Verification items for the finished model (mm, model axes). A direction names the side the tool comes from. Coordinates: 2 decimals unless noted, no trailing zeros. Write each loop counter-clockwise with the first axis right and the second up, starting at its lowest first coordinate (ties: lowest second). Pieces come first, ordered by that corner, then holes. Notation, with made-up numbers: M 43,83.5 L 63,83.5 A11 cw 63,91.5 Z; hole C 2.25,-16 d5. An arc over 180 degrees is marked long. One line per item, written item: value.
Autodesk Inventor part; units mm, degrees
ref_plane "YZ Plane" through (0, 0, 0) normal (1, 0, 0) x (0, 1, 0)
ref_plane "XZ Plane" through (0, 0, 0) normal (0, 1, 0) x (-1, 0, 0)
ref_plane "XY Plane" through (0, 0, 0) normal (0, 0, 1) x (1, 0, 0)
sketch "Sketch1" plane through (0, 0, 0) normal (0, 0, 1) x (1, 0, 0)
  line L0 (0, 0) -> (40, 0)
  line L1 (40, 0) -> (40, -15)
  line L2 (40, -15) -> (0, -15)
  line L3 (0, -15) -> (0, 0)
  dimension "d0" = 40
  dimension "d1" = 15
extrude "Extrusion1" add sketch "Sketch1" along normal blind 5
sketch "Sketch2" plane through (0, 0, 5) normal (0, 0, 1) x (1, 0, 0)
  line L0 (40, 0) -> (0, 0)
  line L1 (5, 0) -> (35, 0)
  line L2 (35, 0) -> (35, -15)
  line L3 (35, -15) -> (5, -15)
  line L4 (5, -15) -> (5, 0)
  line L5 (0, 0) -> (0, -15)
  dimension "d4" = 30
  dimension "d5" = 15
  dimension "d6" = 5
extrude "Extrusion2" add sketch "Sketch2" along normal blind 3
fillet "Fillet1" radius 2 4 edges at (35, -7.5, 5) (35, -7.5, 8) (5, -7.5, 5) (5, -7.5, 8)
sketch "Sketch3" plane through (0, 0, 0) normal (0, 0, -1) x (-1, 0, 0)
  line L0 (0, 0) -> (0, -15)
  line L1 (-40, 0) -> (0, 0)
  line L2 (0, -15) -> (-5, -15)
  line L3 (-5, -15) -> (-5, 0)
  line L4 (-5, 0) -> (0, 0)
  line L5 (0, 0) -> (0, -15)
  line L6 (-40, -15) -> (-40, 0)
  line L7 (0, -15) -> (-40, -15)
  line L8 (-40, 0) -> (-35, 0)
  line L9 (-35, 0) -> (-35, -15)
  line L10 (-35, -15) -> (-40, -15)
  line L11 (-40, -15) -> (-40, 0)
  dimension "d10" = 5
  dimension "d11" = 5
extrude "Extrusion3" add sketch "Sketch3" along normal blind 33.5 contours L0 L2 L3 L1 | L9 L7 L6 L1
sketch "Sketch4" plane through (0, 0, -33.5) normal (0, 0, -1) x (-1, 0, 0)
  line L0 (-35, 0) -> (-35, -15)
  line L1 (-35, -15) -> (-50, -15)
  line L2 (-50, -15) -> (-50, 5)
  line L3 (-50, 5) -> (-35, 5)
  line L4 (-35, 5) -> (-35, -15)
  line L5 (-5, -15) -> (-35, -15)
  line L6 (-5, -15) -> (10, -15)
  line L7 (10, -15) -> (10, 5)
  line L8 (10, 5) -> (-5, 5)
  line L9 (-5, 5) -> (-5, -15)
  point P0 (-4.9365, 0)
  dimension "d18" = 15
  dimension "d19" = 20
  dimension "d20" = 15
extrude "Extrusion4" add sketch "Sketch4" against normal blind 4
fillet "Fillet2" radius 3 6 edges at (0, 0, -12.25) (0, -7.5, 5) (0, -15, -12.25) (40, -15, -12.25) (40, -7.5, 5) (40, 0, -12.25)
fillet "Fillet3" radius 2 6 edges at (-10, 5, -31.5) (5, 5, -31.5) (-10, -15, -31.5) (35, 5, -31.5) (50, 5, -31.5) (50, -15, -31.5)
sketch "Sketch5" plane through (6.873, -15, 8) normal (0, -1, 0) x (1, 0, 0)
  arc A0 (2.2162, 0) -> (7.038, 0) centre (4.6271, -3.5) ccw
  arc A1 (19.2162, 0) -> (24.038, 0) centre (21.6271, -3.5) ccw
  line L0 (-1.8729, -41.5) -> (-14.8729, -41.5)
  line L1 (-14.8729, -37.5) -> (-3.8729, -37.5)
  line L2 (-16.8729, -37.5) -> (-16.8729, -41.5)
  line L3 (-6.8729, -6) -> (-6.8729, -37.5)
  arc A2 (0.0001, 0) -> (-1.9364, -1.5) centre (0.0001, -2) ccw
  arc A3 (-3.8729, -3) -> (-1.9364, -1.5) centre (-3.8729, -1) ccw
  arc A4 (-3.8729, -3) -> (-6.8729, -6) centre (-3.8729, -6) ccw
  line L4 (0, 0) -> (26.254, 0)
  point P0 (-6.873, -8)
  point P1 (-1.8729, -43)
extrude "Extrusion5" cut sketch "Sketch5" against normal blind 1
sketch "Sketch6" plane through (5, -15, 0) normal (0, -1, 0) x (1, 0, 0)
  arc A0 (21.0892, 8) -> (25.911, 8) centre (23.5001, 4.5) ccw
  circle A1 centre (23.5001, 4.5) radius 0.75
  arc A2 (4.0892, 8) -> (8.911, 8) centre (6.5001, 4.5) ccw
  circle A3 centre (6.5001, 4.5) radius 0.75
  point P0 (-5, 0)
  dimension "d27" = 1.5
  dimension "d28" = 1.5
extrude "Extrusion6" cut sketch "Sketch6" against normal blind 10
properties part number "podstawa 01-3"
Item 1: Access from +Z, -Z, +X, -X, +Y, -Y to the whole of each face (thin tool, end or side, straight path). Record for faces 1 (the face through (39.14, -14.1, -12.49)), 2 (the face through (5, -6, -17)), 3 (the face through (4.43, 4.4, -31.47)), 4 (the face through (11.5, -5, 4.5)).
The answers:
face 1: +Z, +X, -Y
face 2: -Z, +Y, -Y
face 3: +Z, -Z, +Y
face 4: -Y
Item 2: Cross-section at A-A, the plane z = -28. Enter the section's corners in (x, y).
The answers:
outline: M 0,-12 A3 ccw 3,-15 L 5,-15 L 5,0 L 3,0 A3 ccw 0,-3 Z; M 35,-15 L 37,-15 A3 ccw 40,-12 L 40,-3 A3 ccw 37,0 L 35,0 Z
Item 3: Draft check along Z on faces 5 (the face through (27.75, -9.56, 4.53)), 6 (the face through (4.2, -7.4, 5.4)), 7 (the face through (28.349, -14.507, 0.253)), 8 (the face through (21.2, 0, 0.3)). Enter one of: released by +Z, released by -Z, zero draft, split by the parting line, or undercut.
The answers:
face 5: undercut
face 6: released by +Z
face 7: undercut
face 8: zero draft
Item 4: Go/stop test with flat-tipped pins: P1, Ø7.5, axis at x = 11.5, z = 4.5, coming from the +Y side; P2, Ø10, axis at y = -8.5, z = -11, coming from the -X side; P3, Ø2.5, axis at x = 28.5, z = 4.5, coming from the -Y side; P4, Ø17, axis at x = 22.5, z = -9.5, coming from the +Y side. Record where each tip stops, or that it passes through.
The answers:
P1: stops at y = 0
P2: stops at x = 0
P3: stops at y = -14
P4: passes through
Item 5: Cross-section at C-C, the plane x = 43. Enter the section's corners in (y, z).
The answers:
outline: M -15,-33.5 L 5,-33.5 L 5,-29.5 L -15,-29.5 Z
Item 6: Scan lines: line 1 (Z direction, x = 11.5, y = -10.75); line 2 (X direction, y = -8.75, z = -23); line 3 (Z direction, x = 16, y = -10.25). Record each from-to range of solid material in increasing order.
The answers:
line 1: z = 0 to 3.75, 5.25 to 8
line 2: x = 0 to 5, 35 to 40
line 3: z = 0 to 8
Item 7: Cross-section at B-B, the plane y = -6. Give the number of separate pieces and of enclosed holes in the cut face, and give its area (3 significant figures).
The answers:
separate pieces: 1
enclosed holes: 2
area: 698 mm²
